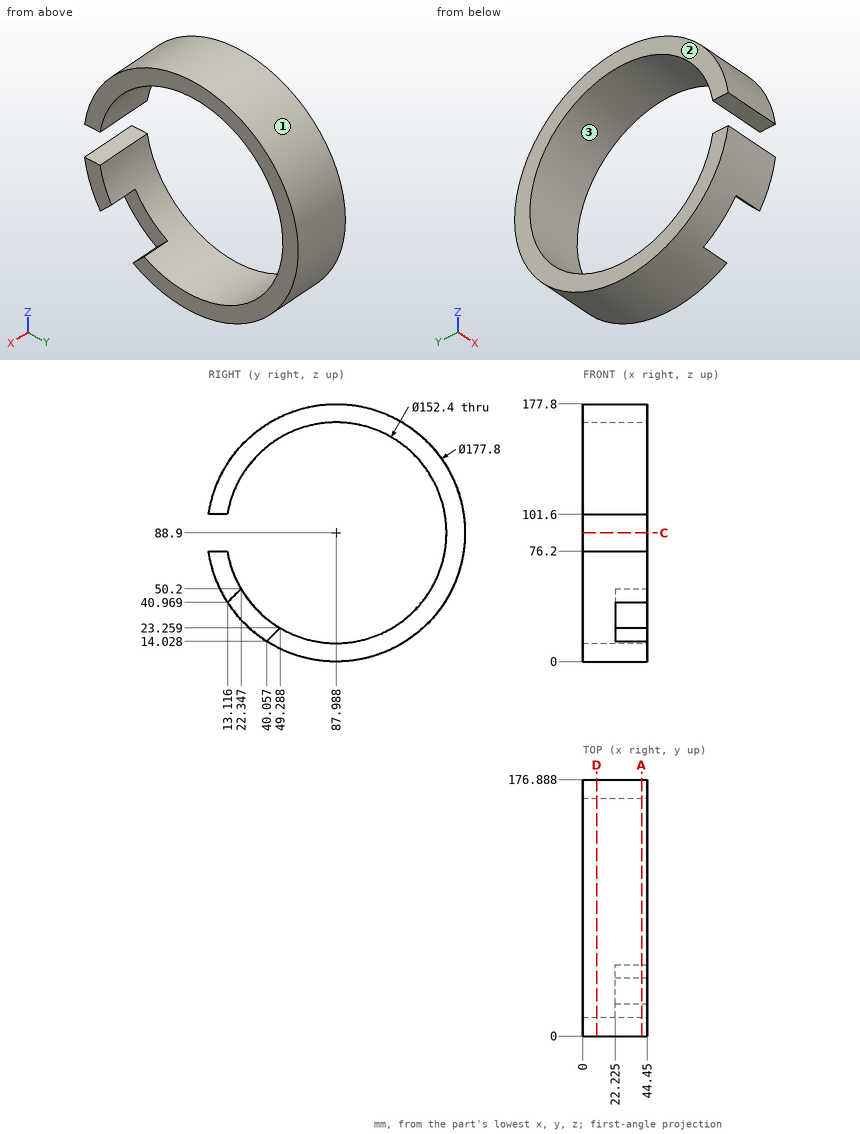
Input: dimensioned drawing with shaded views. Units: mm. Origin: part minimum x, y, z. Coordinates: 2 decimals unless noted, no trailing zeros. Loops run counter-clockwise (first coordinate to the right, second up) from the corner with the lowest first, then second, coordinate; pieces in that order, holes last. Notation, with made-up numbers: M -34.75,77.5 L 24.25,77.5 A25 ccw 24.25,116.5 Z; hole C -7.5,-5 d10. An arc over 180 degrees is marked long. One line per item, written item: value. Start each with the question number.
1) Draft query along Y for the marked faces 1, 2 and 3. Return one class per face: released by +Y, released by -Y, zero draft, split by the parting line, or undercut.
2) Cut plane A-A (x = 40.5). Return loops of the section in (y, z), then the cut area to 4 significant figures.
3) Cut plane C-C (z = 88.9). Return loops of the section in (x, y).
4) Pin query (flat end, axial travel): P1, Ø4, axis at x = 28.5, z = 62, coming from the -Y side; P2, Ø1, axis at x = 34, y = 106.5, coming from the -Z side; P3, Ø2, axis at x = 15.5, z = 153.5, coming from the +Y side. Return the tip coordinate at first contact, or that it passes through.
5) Cut plane D-D (x = 9.5). Return loops of the section in (y, z), then the cut area to 3 significant figures.
6) Material intervals for L1, parallel to Y at x = 29, z = 88; L2, parallel to Z at x = 16.5, y = 123 (1 decimal); L3, parallel to Z at x = 13, y = 23 (1 decimal), sorted ascending. Write a range as from..to.
Evaluation:
1. face 1: split by the parting line
1. face 2: zero draft
1. face 3: undercut
2. outline: M 0,76.2 A88.9 ccw 13.12,40.97 L 22.35,50.2 A76.2 cw 12.85,76.2 Z; M 0,101.6 L 12.85,101.6 A76.2 cw long 49.29,23.26 L 40.06,14.03 A88.9 ccw long Z
2. area: 5,775 mm^2
3. outline: M 0,164.19 L 44.45,164.19 L 44.45,176.89 L 0,176.89 Z
4. P1: y = 2.65
4. P2: z = 1.84
4. P3: y = 150.1
5. outline: M 0,76.2 A88.9 ccw long 0,101.6 L 12.85,101.6 A76.2 cw long 12.85,76.2 Z
5. area: 6,260 mm^2
6. L1: 164.18..176.88
6. L2: 7.2..21.2, 156.6..170.6
6. L3: 28.2..49.1, 128.7..149.6
